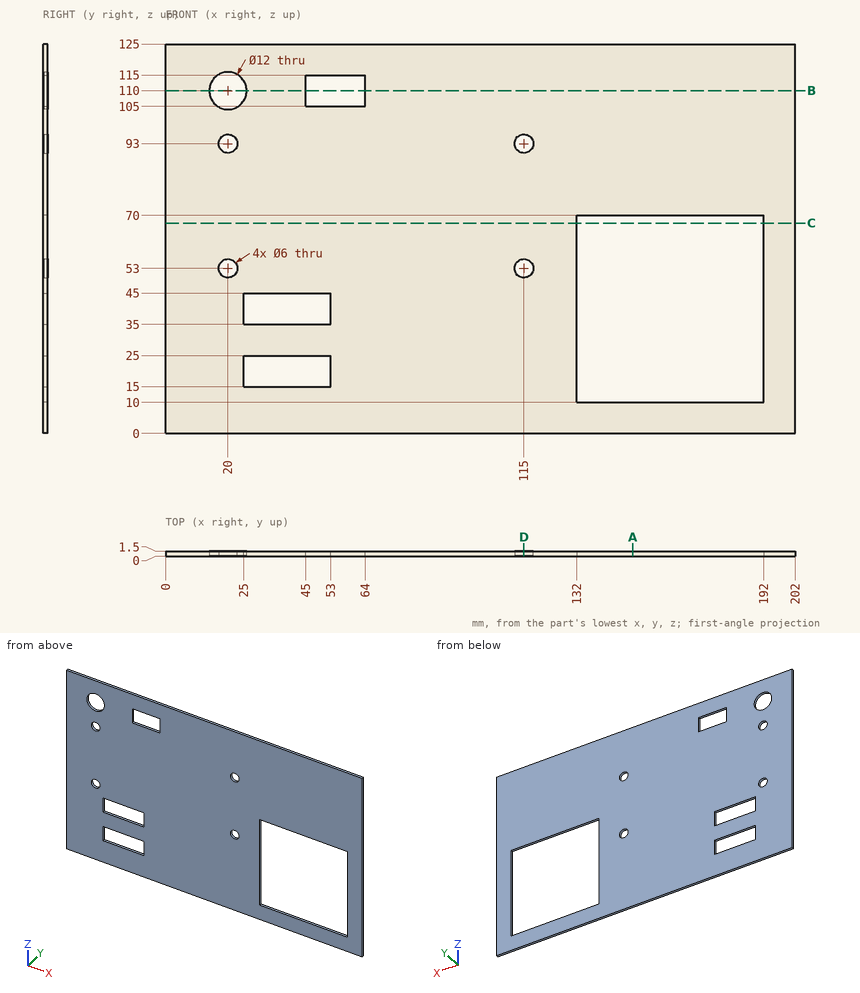
Source: three-view drawing plus pictorial views. Frame: mm from the lowest corner of the part. Give positions to 0.01 mm unless a question says otherwise; leave off trailing zeros. Order: outer loops, then holes, each group sorted by start corner. A loop starts at its lowest first (then second) coordinate and runs counter-clockwise, first axis right, second up. Notation, with made-up numbers: (55.5, -15.5) - (72.5, -15.5) arc R16 cw to (72.5, 10.5) - close; hole circle Ø7 at (68, 82). An arc over 180 degrees is marked (long way). Answer as a JSON object with one key per item and string values. Group by question number.
Q1. Cut plane B-B, the plane z = 110. Output: boundary loops of the cut face in (x, y), then the cut area to 4 significant figures.
Q2. Cut plane C-C, the plane z = 67.5. Output: boundary loops of the cut face in (x, y), then the cut area to 3 significant figures.
Q3. Line query: probe 1 along Z at (x, y) = (20, 1.1); probe 2 along X at (y, z) = (0.9, 24.5); probe 3 along Z at (x, y) = (115, 1). Output: solid intervals per line, ascending.
Q4. Cut plane A-A, the plane x = 150. Output: boundary loops of the cut face in (y, z), then the cut area to 3 significant figures.
Q5. Cut plane D-D, the plane x = 115. Output: boundary loops of the cut face in (y, z).
Results:
{
 "1": {"outline": "(0, 0) - (14, 0) - (14, 1.5) - (0, 1.5) - close; (26, 0) - (45, 0) - (45, 1.5) - (26, 1.5) - close; (64, 0) - (202, 0) - (202, 1.5) - (64, 1.5) - close", "area": "256.5 mm^2"},
 "2": {"outline": "(0, 0) - (132, 0) - (132, 1.5) - (0, 1.5) - close; (192, 0) - (202, 0) - (202, 1.5) - (192, 1.5) - close", "area": "213 mm^2"},
 "3": {"probe 1": "0 to 50, 56 to 90, 96 to 104, 116 to 125", "probe 2": "0 to 25, 53 to 132, 192 to 202", "probe 3": "0 to 50, 56 to 90, 96 to 125"},
 "4": {"outline": "(0, 0) - (1.5, 0) - (1.5, 10) - (0, 10) - close; (0, 70) - (1.5, 70) - (1.5, 125) - (0, 125) - close", "area": "97.5 mm^2"},
 "5": {"outline": "(0, 0) - (1.5, 0) - (1.5, 50) - (0, 50) - close; (0, 56) - (1.5, 56) - (1.5, 90) - (0, 90) - close; (0, 96) - (1.5, 96) - (1.5, 125) - (0, 125) - close"}
}
